Work out the finished part from the listing and answer in its coordinate system (mm). Face numbers are marked on the shaded views. A direction names the side the tool comes from. Coordinates: 2 decimals unless noted, no trailing zeros. Order: outer loops, then holes, each group sorted by start corner. A loop starts at its lowest first (then second) coordinate and runs counter-clockwise, first axis right, second up.
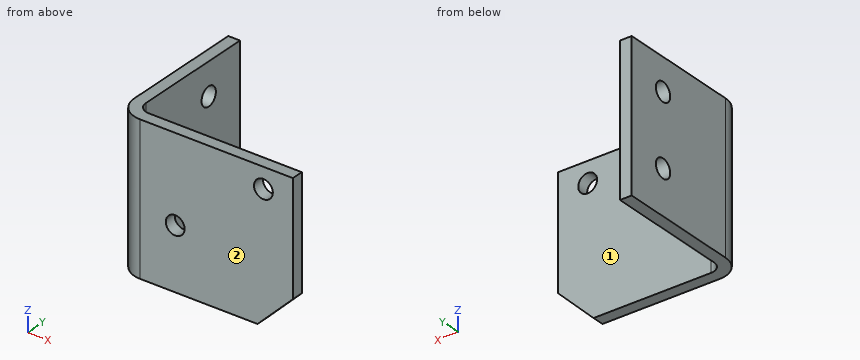
```python
from build123d import *

# Parameters (mm, degrees)
SKETCH5_W                    = 25
SKETCH5_H                    = 25
BASE_FLANGE1_DEPTH           = 2
EDGE_FLANGE1_STRIP_W         = 12
EDGE_FLANGE1_STRIP_H         = 2
EDGE_FLANGE1_STRIP_CUT_DEPTH = 25
EDGE_FLANGE1_DEPTH           = 25
BREAK_CORNER1_START          = 34.648232278
BREAK_CORNER1_OUTLINE_W      = 11
BREAK_CORNER1_OUTLINE_H      = 2
BREAK_CORNER1_DEPTH          = 4.242640687
F_3_2_3_2_DIAMETER_HOLE1_D   = 3.2
F_3_2_3_2_DIAMETER_HOLE2_D   = 3.2


# Read off the part's stored shape, not the designer's step: Break-Corner1
# Sheet-metal steps are written as plain solids
with BuildPart() as part:
    # Sketch5 → Base-Flange1 (new body)
    with BuildSketch(Plane(origin=(0, 0, 0), x_dir=(0, 0, -1), z_dir=(1, 0, 0))):
        with Locations((12.5, 12.5)):
            Rectangle(SKETCH5_W, SKETCH5_H)
    extrude(amount=BASE_FLANGE1_DEPTH)

    # Edge-Flange1 strip (across the edge) → Edge-Flange1 strip cut (cut)
    with BuildSketch(Plane(origin=(2, 0, 0), x_dir=(0, 1, 0), z_dir=(0, 0, -1))):
        with Locations((-2, -1)):
            Rectangle(EDGE_FLANGE1_STRIP_W, EDGE_FLANGE1_STRIP_H)
    extrude(amount=EDGE_FLANGE1_STRIP_CUT_DEPTH, mode=Mode.SUBTRACT)

    # Edge-Flange1 section (across the edge) → Edge-Flange1 (add)
    with BuildSketch(Plane(origin=(2, 0, 0), x_dir=(0, 1, 0), z_dir=(0, 0, -1))):
        with BuildLine():
            Line((0, 2), (0, 28))
            Line((0, 28), (2, 28))
            Line((2, 28), (2, 2))
            ThreePointArc((2, 2), (2.585786438, 0.585786438), (4, 0))
            Line((4, 0), (4, -2))
            ThreePointArc((4, -2), (1.171572875, -0.828427125), (0, 2))
        make_face()
    extrude(amount=EDGE_FLANGE1_DEPTH)

    # Break-Corner1 outline → Break-Corner1 (cut)
    with BuildSketch(Plane(origin=(0, 0, 0), x_dir=(0.7071067811865474, 0, 0.7071067811865477), z_dir=(0.7071067811865476, 0, -0.7071067811865476)).offset(BREAK_CORNER1_START)):
        with Locations((3.5, -1)):
            Rectangle(BREAK_CORNER1_OUTLINE_W, BREAK_CORNER1_OUTLINE_H)
    extrude(amount=BREAK_CORNER1_DEPTH, mode=Mode.SUBTRACT)

    # Ø3.2 (3.2) Diameter Hole1 (through all)
    with Locations(Plane(origin=(2, 0, 0), x_dir=(0, 0, -1), z_dir=(1, 0, 0))):
        with Locations((5.5, 18), (17.5, 18)):
            Hole(F_3_2_3_2_DIAMETER_HOLE1_D / 2)

    # Ø3.2 (3.2) Diameter Hole2 (through all)
    with Locations(Plane(origin=(0, 2, 0), x_dir=(1, 0, 0), z_dir=(0, 1, 0))):
        with Locations((10, 14.5), (25, 3.5)):
            Hole(F_3_2_3_2_DIAMETER_HOLE2_D / 2)


solid = part.part
```
1. The part is cut by section D-D (z = -22.75). Determine the outline of the cut face in (x, y), plus the area to 3 significant figures.
2. The part is cut by section B-B (y = 18). Determine the outline of the cut face in (x, z), plus the area to 3 significant figures.
3. The part is cut by section C-C (z = -5.5). Determine the outline of the cut face in (x, y), plus the area to 3 significant figures.
4. The part is cut by section A-A (x = 25). Determine the outline of the cut face in (y, z).
5. Flat-ended cylindrical pins translate along their axes: pin 1 (4 mm diameter, centred on x = 25, z = -3.5, fed in from +Y); pin 2 (6 mm diameter, centred on x = 18.5, z = -11, fed in from -Y); pin 3 (5 mm diameter, centred on y = 18, z = -17.5, fed in from +X). Find the tip coordinate at first contact, or state that the pin passes through.
6. For the marked faces 1 and 2, determine the directions among +Z, -Z, +X, -X, +Y, -Y from which every point of the face is accessible in a straight line to the end or side of a thin tool.
7. Consider probe 1 along Z at (x, y) = (10, 1.4); probe 2 along X at (y, z) = (5.75, -11.25). Determine where each line is inside the solid, lowest interval first.
Worked out:
1. outline: (0, 4) arc R4 ccw to (4, 0) - (26.25, 0) - (26.25, 2) - (4, 2) arc R2 cw to (2, 4) - (2, 25) - (0, 25) - close
1. area: 95.9 mm2
2. outline: (0, -25) - (2, -25) - (2, -19.1) - (0, -19.1) - close; (0, -15.9) - (2, -15.9) - (2, -7.1) - (0, -7.1) - close; (0, -3.9) - (2, -3.9) - (2, 0) - (0, 0) - close
2. area: 37.2 mm2
3. outline: (0, 4) arc R4 ccw to (4, 0) - (30, 0) - (30, 2) - (4, 2) arc R2 cw to (2, 4) - (2, 16.4) - (0, 16.4) - close; (0, 19.6) - (2, 19.6) - (2, 25) - (0, 25) - close
3. area: 97.0 mm2
4. outline: (0, -24) - (2, -24) - (2, -5.1) - (0, -5.1) - close; (0, -1.9) - (2, -1.9) - (2, 0) - (0, 0) - close
5. pin 1: stops at y = 2
5. pin 2: stops at y = 0
5. pin 3: stops at x = 2
6. face 1: +Z, -Z, +X, +Y
6. face 2: +Z, -Z, +X, -X, -Y
7. probe 1: z = -25 to -16.1, -12.9 to 0
7. probe 2: x = 0 to 2
